from build123d import *

# Parameters (mm, degrees)
SKETCH_1_W      = 40
SKETCH_1_H      = 63
SKETCH_1_R      = 1.7
EXTRUDE_1_DEPTH = 5
FILLET_1_R      = 3


with BuildPart() as part:
    # ｽｹｯﾁ1 → ﾎﾞｽ - 押し出し1 (new body)
    with BuildSketch(Plane(origin=(0, 0, 0), x_dir=(1, 0, 0), z_dir=(0, 1, 0))):
        Rectangle(SKETCH_1_W, SKETCH_1_H)
        with Locations((-15, 26.5)):
            Circle(SKETCH_1_R, mode=Mode.SUBTRACT)
        with Locations((0, 26.5)):
            Circle(SKETCH_1_R, mode=Mode.SUBTRACT)
        with Locations((15, 26.5)):
            Circle(SKETCH_1_R, mode=Mode.SUBTRACT)
        with Locations((0, 11.5)):
            Circle(SKETCH_1_R, mode=Mode.SUBTRACT)
        with Locations((-15, 11.5)):
            Circle(SKETCH_1_R, mode=Mode.SUBTRACT)
        with Locations((15, 11.5)):
            Circle(SKETCH_1_R, mode=Mode.SUBTRACT)
        with Locations((-15, -11.5)):
            Circle(SKETCH_1_R, mode=Mode.SUBTRACT)
        with Locations((0, -11.5)):
            Circle(SKETCH_1_R, mode=Mode.SUBTRACT)
        with Locations((15, -11.5)):
            Circle(SKETCH_1_R, mode=Mode.SUBTRACT)
        with Locations((-15, -26.5)):
            Circle(SKETCH_1_R, mode=Mode.SUBTRACT)
        with Locations((0, -26.5)):
            Circle(SKETCH_1_R, mode=Mode.SUBTRACT)
        with Locations((15, -26.5)):
            Circle(SKETCH_1_R, mode=Mode.SUBTRACT)
    extrude(amount=EXTRUDE_1_DEPTH)

    # ﾌｨﾚｯﾄ1
    fillet_1_edges = [part.edges().sort_by_distance(p)[0] for p in [
        (20, 2.5, 31.5),
        (-20, 2.5, 31.5),
        (-20, 2.5, -31.5),
        (20, 2.5, -31.5),
    ]]
    fillet(fillet_1_edges, radius=FILLET_1_R)


solid = part.part
Input: part model. Units: mm. Frame: model coordinates. Round coordinates to 2 decimals unless told otherwise and drop trailing zeros. Order: outer loops, then holes, each group sorted by start corner. A loop starts at its lowest first (then second) coordinate and runs counter-clockwise, first axis right, second up. Notation, with made-up numbers: (15, 6) - (51, 6) arc R32 ccw to (51, 43) - close; hole circle Ø1 at (68.5, 1.5). An arc over 180 degrees is marked (long way). Answer as a JSON object with one key per item and string values. Group by question number.
(1) Draft query along Z for faces 1 (the face through (19.1, 2.54, 30.64)), 2 (the face through (19.1, 2.54, -30.64)), 3 (the face through (-13.43, 2.46, 12.15)). Return one class per face: released by +Z, released by -Z, zero draft, split by the parting line, or undercut.
(2) Cut plane C-C (y = 2.3). Count the separate pieces of the cut face and the enclosed holes in it, then the cut area to 3 significant figures.
(3) Cut plane B-B (x = -15). Return loops of the section in (y, z), then the cut area to 3 significant figures.
(4) Material intervals for probe 1 along X at (y, z) = (1.6, 11.5); probe 2 along Z at (x, y) = (0, 3.85); probe 3 along Z at (x, y) = (13.5, 3.2), sorted ascending. Write a range as from..to.
(5) Cut plane A-A (z = -26.5). Return loops of the section in (x, y).
(6) Cut plane D-D (x = -1). Return loops of the section in (y, z), then the cut area to 3 significant figures.
Here are the results:
{
 "1": {"face 1": "released by +Z", "face 2": "released by -Z", "face 3": "undercut"},
 "2": {"separate pieces": "1", "enclosed holes": "12", "area": "2,400 mm^2"},
 "3": {"outline": "(0, -31.5) - (5, -31.5) - (5, -28.2) - (0, -28.2) - close; (0, -24.8) - (5, -24.8) - (5, -13.2) - (0, -13.2) - close; (0, -9.8) - (5, -9.8) - (5, 9.8) - (0, 9.8) - close; (0, 13.2) - (5, 13.2) - (5, 24.8) - (0, 24.8) - close; (0, 28.2) - (5, 28.2) - (5, 31.5) - (0, 31.5) - close", "area": "247 mm^2"},
 "4": {"probe 1": "x = -20..-16.7, -13.3..-1.7, 1.7..13.3, 16.7..20", "probe 2": "z = -31.5..-28.2, -24.8..-13.2, -9.8..9.8, 13.2..24.8, 28.2..31.5", "probe 3": "z = -31.5..-27.3, -25.7..-12.3, -10.7..10.7, 12.3..25.7, 27.3..31.5"},
 "5": {"outline": "(-20, 0) - (-16.7, 0) - (-16.7, 5) - (-20, 5) - close; (-13.3, 0) - (-1.7, 0) - (-1.7, 5) - (-13.3, 5) - close; (1.7, 0) - (13.3, 0) - (13.3, 5) - (1.7, 5) - close; (16.7, 0) - (20, 0) - (20, 5) - (16.7, 5) - close"},
 "6": {"outline": "(0, -31.5) - (5, -31.5) - (5, -27.87) - (0, -27.87) - close; (0, -25.13) - (5, -25.13) - (5, -12.87) - (0, -12.87) - close; (0, -10.13) - (5, -10.13) - (5, 10.13) - (0, 10.13) - close; (0, 12.87) - (5, 12.87) - (5, 25.13) - (0, 25.13) - close; (0, 27.87) - (5, 27.87) - (5, 31.5) - (0, 31.5) - close", "area": "260 mm^2"}
}
